Build history of the part. All positions in model axes, mm. Face numbers are marked on the shaded views. A direction names the side the tool comes from. Coordinates: 2 decimals unless noted, no trailing zeros. Loops run counter-clockwise (first coordinate to the right, second up) from the corner with the lowest first, then second, coordinate; pieces in that order, holes last.
(1) Wall check: L1, parallel to X at y = 9.25, z = -16; L2, parallel to Z at x = 19.5, y = 19; L3, parallel to Z at x = -6.5, y = 6. Give the ranges that are in metal, low to high.
(2) Flat gauge pins, fed straight in: P1, Ø8, axis at y = 4, z = -4.5, coming from the +X side; P2, Ø8, axis at y = 14, z = -1, coming from the -X side; P3, Ø1, axis at y = 8.5, z = -15.5, coming from the +X side; P4, Ø3, axis at x = -33, z = 1, coming from the -Y side. Where does each tip first touch, or does it go through?
(3) Slice it at D-D (z = 24). Give the cut face in (x, y), and give its area (3 significant figures).
(4) Slice it at B-B (z = -20). Give the cut face in (x, y).
(5) Two-plate mould, pull along Z, no slides. Class the marked faces 3, 4 and 5: pulls with the +Z half, pulls with the -Z half, needs draft (parallel to the pull), parting line crosses it, or undercut.
(6) Tool access for the marked faces 1 and 2: list every direction of +Z, -Z, +X, -X, +Y, -Y with a clear straight run to the whole face (end or side of a thin tool).
(7) Slice it at A-A (x = 21.5). Give the cut face in (y, z), and give its area (3 significant figures).
(8) Slice it at C-C (x = -31). Give the cut face in (y, z), and give its area (3 significant figures).
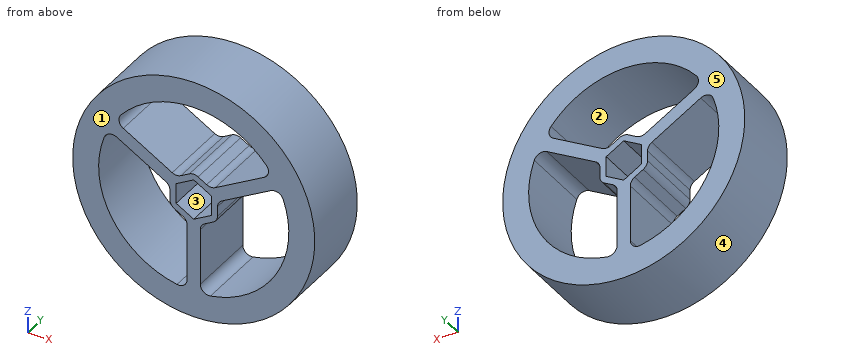
from build123d import *

# Parameters (mm, degrees)
SKETCH1_R           = 44.45
BOSS_EXTRUDE1_DEPTH = 25.4
FILLET1_R           = 3.175


with BuildPart() as part:
    # Sketch1 → Boss-Extrude1 (new body)
    with BuildSketch(Plane(origin=(0, 0, 0), x_dir=(1, 0, 0), z_dir=(0, 1, 0))):
        with Locations(Location((0, 0, 0), (0, 0, 270))):
            Circle(SKETCH1_R)
        Polygon((-6.4516, 3.724832997), (0, 7.449665993), (6.4516, 3.724832997), (6.4516, -3.724832997), (0, -7.449665993), (-6.4516, -3.724832997), align=None, mode=Mode.SUBTRACT)
        with BuildLine():
            Line((2.413, 8.696165225), (2.413, 34.841542101))
            ThreePointArc((2.413, 34.841542101), (30.245937227, 17.4625), (31.380160567, -15.331051751))
            Line((31.380160567, -15.331051751), (8.7376, -2.258363313))
            Line((8.7376, -2.258363313), (8.7376, 5.044655712))
            Line((8.7376, 5.044655712), (2.413, 8.696165225))
        make_face(mode=Mode.SUBTRACT)
        with BuildLine():
            Line((-2.413, 34.841542101), (-2.413, 8.696165225))
            Line((-2.413, 8.696165225), (-8.7376, 5.044655712))
            Line((-8.7376, 5.044655712), (-8.7376, -2.258363313))
            Line((-8.7376, -2.258363313), (-31.380160567, -15.331051751))
            ThreePointArc((-31.380160567, -15.331051751), (-30.245937227, 17.4625), (-2.413, 34.841542101))
        make_face(mode=Mode.SUBTRACT)
        with BuildLine():
            Line((-28.967160567, -19.51049035), (-6.3246, -6.437801912))
            Line((-6.3246, -6.437801912), (0, -10.089311424))
            Line((0, -10.089311424), (6.3246, -6.437801912))
            Line((6.3246, -6.437801912), (28.967160567, -19.51049035))
            ThreePointArc((28.967160567, -19.51049035), (0, -34.925), (-28.967160567, -19.51049035))
        make_face(mode=Mode.SUBTRACT)
    extrude(amount=BOSS_EXTRUDE1_DEPTH)

    # Fillet1
    fillet1_edges = [part.edges().sort_by_distance(p)[0] for p in [
        (-8.7376, 12.7, -5.044655712),
        (-2.413, 12.7, -8.696165225),
        (-2.413, 12.7, -34.841542101),
        (-31.380160567, 12.7, 15.331051751),
        (-8.7376, 12.7, 2.258363313),
        (31.380160567, 12.7, 15.331051751),
        (2.413, 12.7, -34.841542101),
        (2.413, 12.7, -8.696165225),
        (8.7376, 12.7, -5.044655712),
        (8.7376, 12.7, 2.258363313),
        (-28.967160567, 12.7, 19.51049035),
        (28.967160567, 12.7, 19.51049035),
        (6.3246, 12.7, 6.437801912),
        (0, 12.7, 10.089311424),
        (-6.3246, 12.7, 6.437801912),
    ]]
    fillet(fillet1_edges, radius=FILLET1_R)


solid = part.part
Response values:
1. L1: x = -41.47 to -31.04, -2.41 to 2.41, 31.04 to 41.47
1. L2: z = -39.94 to -28.97, 8.47 to 14.04, 28.97 to 39.94
1. L3: z = -43.97 to -34.31, -6.34 to 6.93, 34.31 to 43.97
2. P1: stops at x = 44.45
2. P2: stops at x = -44.45
2. P3: stops at x = 41.84
2. P4: passes through
3. outline: (-37.41, 0) - (-25.37, 0) - (-25.37, 25.4) - (-37.41, 25.4) - close; (25.37, 0) - (37.41, 0) - (37.41, 25.4) - (25.37, 25.4) - close
3. area: 612 mm2
4. outline: (-39.7, 0) - (-28.63, 0) - (-28.63, 25.4) - (-39.7, 25.4) - close; (-2.41, 0) - (2.41, 0) - (2.41, 25.4) - (-2.41, 25.4) - close; (28.63, 0) - (39.7, 0) - (39.7, 25.4) - (28.63, 25.4) - close
5. face 3: undercut
5. face 4: parting line crosses it
5. face 5: needs draft
6. face 1: +Z, -Z, +X, -X, -Y
6. face 2: +Y, -Y
7. outline: (0, -38.9) - (25.4, -38.9) - (25.4, -27.52) - (0, -27.52) - close; (0, 9.63) - (25.4, 9.63) - (25.4, 15.2) - (0, 15.2) - close; (0, 27.52) - (25.4, 27.52) - (25.4, 38.9) - (0, 38.9) - close
7. area: 720 mm2
8. outline: (0, -31.86) - (25.4, -31.86) - (25.4, -16.09) - (0, -16.09) - close; (0, 13.75) - (25.4, 13.75) - (25.4, 31.86) - (0, 31.86) - close
8. area: 860 mm2
